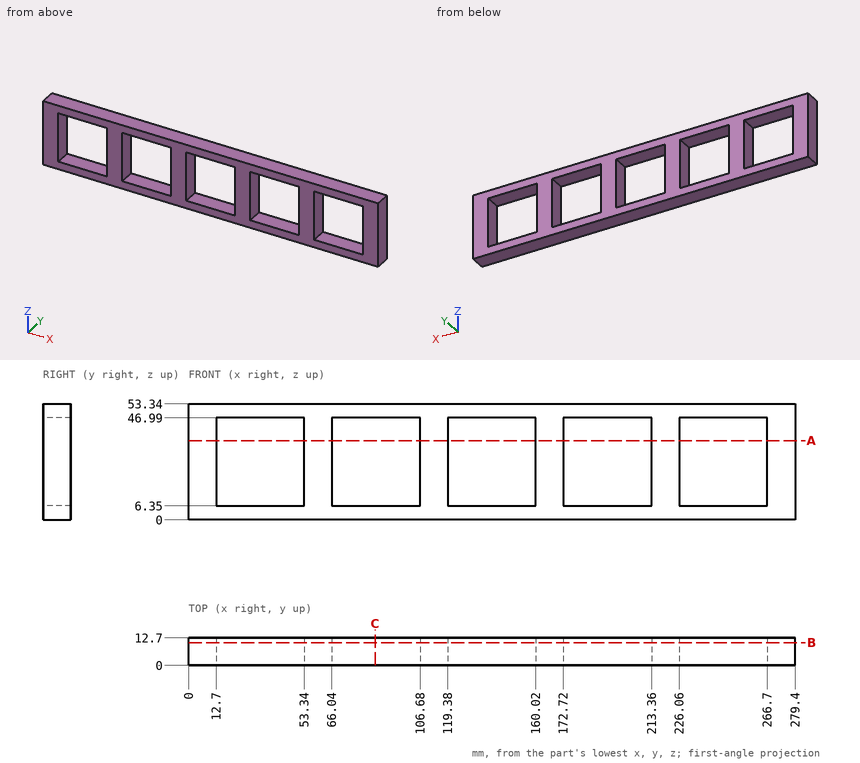
For this review, use the dimensioned drawing (mm, ordinates from the lowest corner) and the shaded views. Round coordinates to 2 decimals unless told otherwise and drop trailing zeros. Order: outer loops, then holes, each group sorted by start corner. A loop starts at its lowest first (then second) coordinate and runs counter-clockwise, first axis right, second up.
1) Consider section B-B (y = 10.5). State the section outline as (x, z) points, plus the area to 3 significant figures.
The answers:
outline: (0, 0) - (279.4, 0) - (279.4, 53.34) - (0, 53.34) - close; hole (12.7, 6.35) - (53.34, 6.35) - (53.34, 46.99) - (12.7, 46.99) - close; hole (66.04, 6.35) - (106.68, 6.35) - (106.68, 46.99) - (66.04, 46.99) - close; hole (119.38, 6.35) - (160.02, 6.35) - (160.02, 46.99) - (119.38, 46.99) - close; hole (172.72, 6.35) - (213.36, 6.35) - (213.36, 46.99) - (172.72, 46.99) - close; hole (226.06, 6.35) - (266.7, 6.35) - (266.7, 46.99) - (226.06, 46.99) - close
area: 6,650 mm2
2) Consider section A-A (z = 36.5). State the section outline as (x, y) points.
The answers:
outline: (0, 0) - (12.7, 0) - (12.7, 12.7) - (0, 12.7) - close; (53.34, 0) - (66.04, 0) - (66.04, 12.7) - (53.34, 12.7) - close; (106.68, 0) - (119.38, 0) - (119.38, 12.7) - (106.68, 12.7) - close; (160.02, 0) - (172.72, 0) - (172.72, 12.7) - (160.02, 12.7) - close; (213.36, 0) - (226.06, 0) - (226.06, 12.7) - (213.36, 12.7) - close; (266.7, 0) - (279.4, 0) - (279.4, 12.7) - (266.7, 12.7) - close
3) For L1, parallel to X at y = 2.75, z = 24.5; L2, parallel to Z at x = 156, y = 6.5, list the stretches that pass through material, from the lowest coordinate up.
The answers:
L1: x = 0 to 12.7, 53.34 to 66.04, 106.68 to 119.38, 160.02 to 172.72, 213.36 to 226.06, 266.7 to 279.4
L2: z = 0 to 6.35, 46.99 to 53.34
4) Consider section C-C (x = 86). State the section outline as (y, z) points, plus the area to 3 significant figures.
The answers:
outline: (0, 0) - (12.7, 0) - (12.7, 6.35) - (0, 6.35) - close; (0, 46.99) - (12.7, 46.99) - (12.7, 53.34) - (0, 53.34) - close
area: 161 mm2
